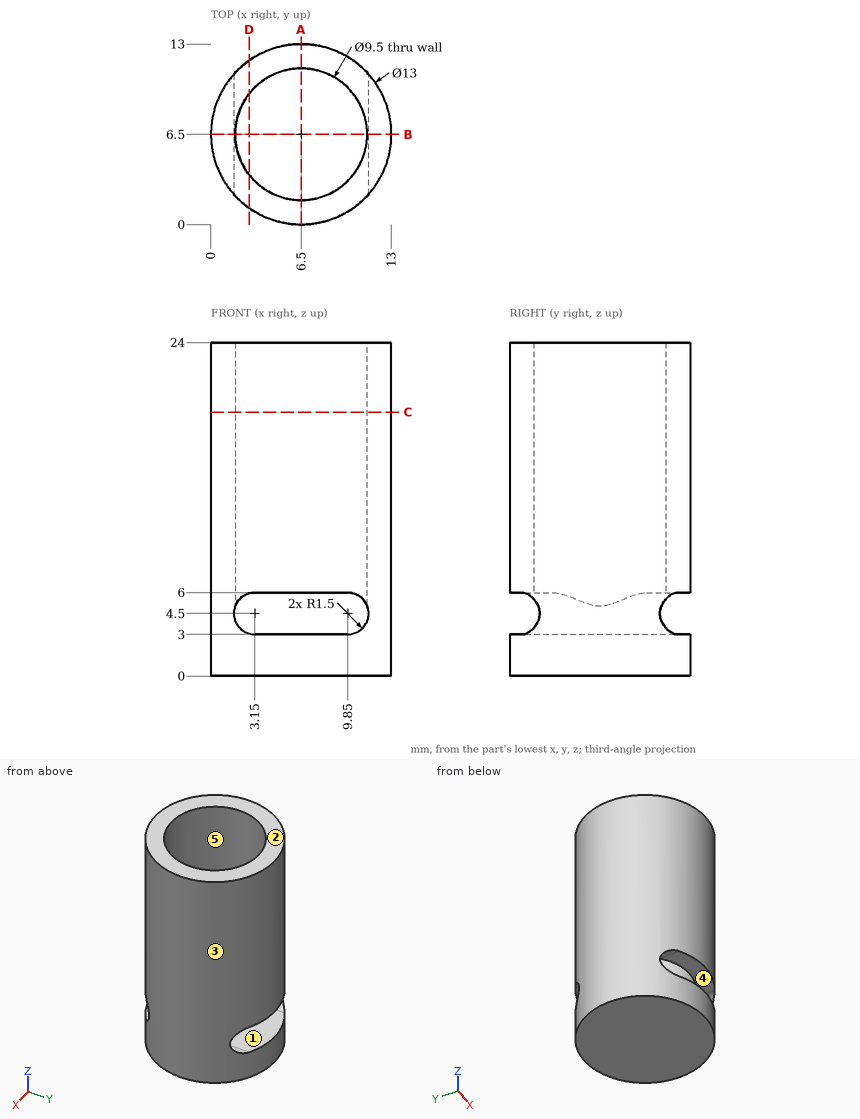
Here's the drawing with two shaded views (mm, measured from the low corner). I have some questions. A direction names the side the tool comes from. Round coordinates to 2 decimals unless told otherwise and drop trailing zeros. Loops run counter-clockwise (first coordinate to the right, second up) from the corner with the lowest first, then second, coordinate; pieces in that order, holes last. Notation, with made-up numbers: (27, 16) - (76, 16) arc R33 cw to (76, 47) - close; hole circle Ø5 at (23, 15). An arc over 180 degrees is marked (long way). Use CSV: the item, a comma, the result in double quotes. Start each with the question number.
1) For the marked faces 1 and 2, which set-ups out of +Z, -Z, +X, -X, +Y, -Y let a thin tool reach every point of the face, with its end or its side?
2) If we section it at A-A on x = 6.5: Write out the boundary of the cut face in (y, z).
3) If we section it at B-B on y = 6.5: Write out the boundary of the cut face in (x, z).
4) If we section it at C-C on z = 19: Write out the boundary of the cut face in (x, y).
5) For pin 1 Ø4 at (x, z) = (2, 8) entering from +Y; pin 2 Ø2 at (x, z) = (8.5, 21.5) entering from -Y; pin 3 Ø6 at (x, z) = (11, 13.5) entering from +Y, each with a flat end and sliding along its axis, tell me the tip position at first contact or that it passes through.
6) We'd pull the mould along Y, two halves only. Please class the marked faces 3, 4 and 5: released by +Y, released by -Y, zero draft, split by the parting line, or undercut.
7) Please list where these lines run through material, in increasing order: probe 1 along Y at (x, z) = (6.5, 14.25); probe 2 along Z at (x, y) = (6.5, 12.5); probe 3 along Z at (x, y) = (8, 4.5). Write a range as [from, to].
8) If we section it at D-D on x = 2.75: Write out the boundary of the cut face in (y, z).
Geometry results:
1,face 1,"+Y, -Y"
1,face 2,"+Z, +X, -X, +Y, -Y"
2,outline,"(0, 0) - (13, 0) - (13, 3) - (0, 3) - close; (0, 6) - (1.75, 6) - (1.75, 24) - (0, 24) - close; (11.25, 6) - (13, 6) - (13, 24) - (11.25, 24) - close"
3,outline,"(0, 0) - (13, 0) - (13, 24) - (11.25, 24) - (11.25, 5.04) arc R1.5 cw to (9.85, 3) - (3.15, 3) arc R1.5 cw to (1.75, 5.04) - (1.75, 24) - (0, 24) - close"
4,outline,"circle Ø13 at (6.5, 6.5); hole circle Ø9.5 at (6.5, 6.5)"
5,pin 1,"stops at y = 12.5"
5,pin 2,"stops at y = 0.08"
5,pin 3,"stops at y = 12.82"
6,face 3,"split by the parting line"
6,face 4,"zero draft"
6,face 5,"undercut"
7,probe 1,"y = [0, 1.75], [11.25, 13]"
7,probe 2,"z = [0, 3], [6, 24]"
7,probe 3,"z = [0, 3]"
8,outline,"(1.19, 0) - (11.81, 0) - (11.81, 3.05) - (1.19, 3.05) - close; (1.19, 5.95) - (3.58, 5.95) - (3.58, 24) - (1.19, 24) - close; (9.42, 5.95) - (11.81, 5.95) - (11.81, 24) - (9.42, 24) - close"
